Read the model definition and answer for the solid it produces. Units are mm, in the model's axes. A direction names the side the tool comes from. Round coordinates to 2 decimals unless told otherwise and drop trailing zeros. Write each loop counter-clockwise with the first axis right and the second up, starting at its lowest first coordinate (ties: lowest second). Pieces come first, ordered by that corner, then holes. Notation, with made-up numbers: (-34, 25.25) - (20, 25.25) arc R20 cw to (20, 48.25) - close; hole circle Ø8 at (48.25, 65). An arc over 180 degrees is marked (long way). Use one line per item in the form item = value. Start each with the question number.
1) The part is cut by section C-C, the plane x = 111. Give the vertices of the cut face in (y, z), plus the area to 3 significant figures.
2) Each of these flat-tipped pins is pushed along its axis until it touches: pin 1 (1 mm diameter, centred on x = 81, z = 1.5, fed in from -Y); pin 2 (2.5 mm diameter, centred on x = -4.5, z = 0, fed in from +Y); pin 3 (3 mm diameter, centred on y = 3, z = 14.5, fed in from -X). Where does it stop, or does it pass through?
3) Consider line 1 along Z through (x, y) = (-3.7, 0); line 2 along Z through (x, y) = (5, 0); line 3 along X through (y, z) = (-1.5, 13). Determine where each line is inside the solid, lowest interval first. Write a range as from..to.
4) The part is cut by section A-A, the plane x = 12.5. Give the vertices of the cut face in (y, z), plus the area to 3 significant figures.
5) The part is cut by section B-B, the plane z = 16. Give the vertices of the cut face in (x, y), plus the area to 3 significant figures.
6) The part is cut by section D-D, the plane y = -17. Give the vertices of the cut face in (x, z), plus the area to 3 significant figures.
7) For a pull along Y with two mould halves and no side action, classify faces 5 (the face through (-6.1, -3, -4)), 6 (the face through (123.67, -4.336, -19.524)), 7 (the face through (15.486, 0.533, 0.221)) as released by +Y, released by -Y, zero draft, split by the parting line, or undercut.
8) For faces 1 (the face through (-4, 5, 0)), 2 (the face through (-4, -5, 0)), 3 (the face through (128.6, 0, 0)), 4 (the face through (6, 3.07, -1.27)), determine the directions among +Z, -Z, +X, -X, +Y, -Y from which every point of the face is accessible in a straight line to the end or side of a thin tool.
Autodesk Inventor part; units mm, degrees
ref_plane "FDT_PIRODACC_F1_XY" through (-6.1, 0, 0) normal (-1, 0, 0) x (0, 1, 0)
ref_plane "FDT_PIRODACC_F1_YZ" through (-6.1, 0, 0) normal (0, 1, 0) x (0, 0, -1)
ref_plane "FDT_PIRODACC_F1_ZX" through (-6.1, 0, 0) normal (0, 0, -1) x (-1, 0, 0)
sketch "Sketch_1" plane through (0, 0, 0) normal (0, 0, 1) x (1, 0, 0)
  line L0 (128.6, 0) -> (-6.1, 0)
  line L1 (-6.1, 0) -> (-6.1, 6)
  line L2 (-6.1, 6) -> (128.6, 6)
  line L3 (128.6, 6) -> (128.6, 0)
  line L4 (128.6, 0) -> (-6.1, 0)
revolve "Revolution1" add sketch "Sketch_1" angle 360 about axis through (128.6, 0, 0) along (1, 0, 0)
sketch "Sketch_11" plane through (0, 0, 0) normal (0, 0, 1) x (1, 0, 0)
  line L0 (128.6, 0) -> (118.6, 0)
  line L1 (118.6, 0) -> (118.6, 20)
  line L2 (118.6, 20) -> (128.6, 20)
  line L3 (128.6, 20) -> (128.6, 0)
  line L4 (128.6, 0) -> (118.6, 0)
revolve "Revolution2" add sketch "Sketch_11" angle 360 about axis through (128.6, 0, 0) along (1, 0, 0)
sketch "Sketch_20" plane through (0, 0, 0) normal (0, 0, 1) x (1, 0, 0)
  line L0 (-36.2, -16) -> (4.9509, -16)
  line L1 (4.9509, -16) -> (-1.4, -5)
  line L2 (-1.4, -5) -> (-6.1, -5)
  line L3 (-6.1, -5) -> (-6.1, -10)
  line L4 (-6.1, -10) -> (-30.1, -10)
  line L5 (-30.1, -10) -> (-30.1, 10)
  line L6 (-30.1, 10) -> (-6.1, 10)
  line L7 (-6.1, 10) -> (-6.1, 5)
  line L8 (-6.1, 5) -> (-1.4, 5)
  line L9 (-1.4, 5) -> (4.9509, 16)
  line L10 (4.9509, 16) -> (-36.2, 16)
  line L11 (-36.2, 16) -> (-36.2, -16)
extrude "Extrusion1" cut sketch "Sketch_20" along normal mid plane 24
sketch "Sketch_2" plane through (0, 0, 0) normal (0, 0, 1) x (1, 0, 0)
  line L0 (15.8188, 0) -> (-6.1, 0)
  line L1 (-6.1, 0) -> (-6.1, 4.6)
  line L2 (-6.1, 4.6) -> (-5.7, 4.2)
  line L3 (-5.7, 4.2) -> (-2.8, 4.2)
  line L4 (-2.8, 4.2) -> (-2.8, 4)
  line L5 (-2.8, 4) -> (-2.1235, 3.3235)
  line L6 (-2.1235, 3.3235) -> (13.9, 3.3235)
  line L7 (13.9, 3.3235) -> (15.8188, 0)
  line L8 (15.8188, 0) -> (-6.1, 0)
revolve "Revolution3" cut sketch "Sketch_2" angle 360 about axis through (15.8188, 0, 0) along (1, 0, 0)
thread "Thread1"
ref_plane "FDT_PIRODACC_F1_XY" through (-6.1, 0, 0) normal (-1, 0, 0) x (0, 1, 0)
ref_plane "FDT_PIRODACC_F1_YZ" through (-6.1, 0, 0) normal (0, 1, 0) x (0, 0, -1)
ref_plane "FDT_PIRODACC_F1_ZX" through (-6.1, 0, 0) normal (0, 0, -1) x (-1, 0, 0)
ref_plane "NUT1_XY" through (-12.6, 0, 0) normal (1, 0, 0) x (0, 0, -1)
ref_plane "NUT1_YZ" through (-12.6, 0, 0) normal (0, 0, -1) x (0, 1, 0)
ref_plane "NUT1_ZX" through (-12.6, 0, 0) normal (0, 1, 0) x (1, 0, 0)
ref_plane "PISTON_XY" through (128.6, 0, 0) normal (1, 0, 0) x (0, 0, -1)
ref_plane "PISTON_YZ" through (128.6, 0, 0) normal (0, 0, -1) x (0, 1, 0)
ref_plane "PISTON_ZX" through (128.6, 0, 0) normal (0, 1, 0) x (1, 0, 0)
properties part number "536288 ADN-100-P-I_(KS)"
Geometry results:
q1.outline = circle Ø12 at (0, 0)
q1.area = 113 mm2
q2.pin_1 = -5.92
q2.pin_2 = 5
q2.pin_3 = 118.6
q3.line_1 = -6..-4.2, 4.2..6
q3.line_2 = -6..-3.32, 3.32..6
q3.line_3 = 118.6..128.6
q4.outline = circle Ø12 at (0, 0); hole circle Ø6.65 at (0, 0)
q4.area = 78.4 mm2
q5.outline = (118.6, -12) - (128.6, -12) - (128.6, 12) - (118.6, 12) - close
q5.area = 240 mm2
q6.outline = (118.6, -10.54) - (128.6, -10.54) - (128.6, 10.54) - (118.6, 10.54) - close
q6.area = 211 mm2
q7.face_5 = zero draft
q7.face_6 = split by the parting line
q7.face_7 = undercut
q8.face_1 = +Z, -Z, -X, +Y
q8.face_2 = +Z, -Z, -X, -Y
q8.face_3 = +Z, -Z, +X, +Y, -Y
q8.face_4 = -X
